CAD build for the part. Positions are in the model's coordinates, mm. Face numbers are marked on the shaded views. Round coordinates to 2 decimals unless told otherwise and drop trailing zeros. Loops run counter-clockwise (first coordinate to the right, second up) from the corner with the lowest first, then second, coordinate; pieces in that order, holes last. Notation, with made-up numbers: (-9, 41) -> (42, 41) arc R27 ccw to (42, 64) -> close; hole circle Ø9 at (-29, 35). An arc over 180 degrees is marked (long way). Answer as CSV lines item,"result".
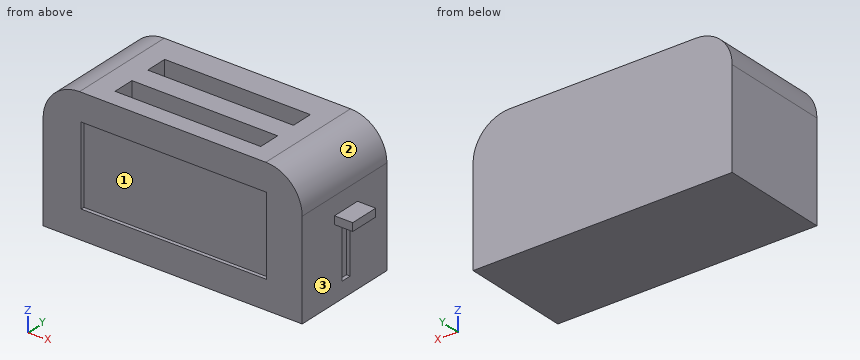
```python
from build123d import *

# Parameters (mm, degrees)
F0_W      = 180.69154
F0_H      = 93.475536
F1_DEPTH  = 76.2
F2_R      = 25.4
F3_W      = 101.6
F3_H      = 15.24
F4_DEPTH  = 76.2
F5_W      = 129.371017
F5_H      = 55.014919
F6_DEPTH  = 2.54
F7_W      = 20.702834
F7_H      = 5.605837
F8_DEPTH  = 12.7
F9_W      = 7.488246
F9_H      = 38.76276
F10_DEPTH = 2.54


with BuildPart() as f1:
    # F0 (on Front) → F1 (new body)
    with BuildSketch(Plane.XZ):
        with Locations((0, -8.763328)):
            Rectangle(F0_W, F0_H)
    extrude(amount=F1_DEPTH)

    # F2
    f2_edges = [f1.edges().sort_by_distance(p)[0] for p in [
        (90.34577, -38.1, 37.97444),
        (-90.34577, -38.1, 37.97444),
    ]]
    fillet(f2_edges, radius=F2_R)

    # F3 (on face) → F4 (cut)
    with BuildSketch(Plane.XY.offset(37.97444)):
        with Locations((1.085338, -56.274154)):
            Rectangle(F3_W, F3_H)
        with Locations((0.680554, -26.320373)):
            Rectangle(F3_W, F3_H)
    extrude(amount=-F4_DEPTH, mode=Mode.SUBTRACT)

    # F5 (on face) → F6 (cut)
    with BuildSketch(Plane.XZ.offset(76.2)):
        with Locations((0.859611, -8.333524)):
            Rectangle(F5_W, F5_H)
    extrude(amount=-F6_DEPTH, mode=Mode.SUBTRACT)

    # F7 (on face) → F8 (join)
    with BuildSketch(Plane.YZ.offset(90.34577)):
        with Locations((-36.778546, -2.802919)):
            Rectangle(F7_W, F7_H)
    extrude(amount=F8_DEPTH)

    # F9 (on face) → F10 (cut)
    with BuildSketch(Plane.YZ.offset(90.34577)):
        with Locations((-36.778546, -24.987215)):
            Rectangle(F9_W, F9_H)
    extrude(amount=-F10_DEPTH, mode=Mode.SUBTRACT)


solid = f1.part
```
Q1. Slice it at A-A, the plane z = 6. Give the cut face in (x, y), and give its area (3 significant figures).
Results:
outline,"(-90.35, -76.2) -> (-63.83, -76.2) -> (-63.83, -73.66) -> (65.55, -73.66) -> (65.55, -76.2) -> (90.35, -76.2) -> (90.35, 0) -> (-90.35, 0) -> close; hole (-50.12, -33.94) -> (51.48, -33.94) -> (51.48, -18.7) -> (-50.12, -18.7) -> close; hole (-49.71, -63.89) -> (51.89, -63.89) -> (51.89, -48.65) -> (-49.71, -48.65) -> close"
area,"10,300 mm2"
Q2. Slice it at B-B, the plane y = -56. Give the cut face in (x, z), and give its area (3 significant figures).
Results:
outline,"(-90.35, -55.5) -> (90.35, -55.5) -> (90.35, 12.57) arc R25.4 ccw to (64.95, 37.97) -> (51.89, 37.97) -> (51.89, -38.23) -> (-49.71, -38.23) -> (-49.71, 37.97) -> (-64.95, 37.97) arc R25.4 ccw to (-90.35, 12.57) -> close"
area,"8,870 mm2"
Q3. Slice it at C-C, the plane x = 17. Give the cut face in (y, z), and give its area (3 significant figures).
Results:
outline,"(-76.2, -55.5) -> (0, -55.5) -> (0, 37.97) -> (-18.7, 37.97) -> (-18.7, -38.23) -> (-33.94, -38.23) -> (-33.94, 37.97) -> (-48.65, 37.97) -> (-48.65, -38.23) -> (-63.89, -38.23) -> (-63.89, 37.97) -> (-76.2, 37.97) -> (-76.2, 19.17) -> (-73.66, 19.17) -> (-73.66, -35.84) -> (-76.2, -35.84) -> close"
area,"4,660 mm2"
Q4. Probe L1, parallel to Y at x = -10, z = 29; L2, parallel to Y at x = -32.5, z = 5; L3, parallel to X at y = -50, z = 4. List the from-to ranges inside material, lowest first. Write a range as [from, to].
Results:
L1,"[-76.2, -63.89], [-48.65, -33.94], [-18.7, 0]"
L2,"[-73.66, -63.89], [-48.65, -33.94], [-18.7, 0]"
L3,"[-90.35, -49.71], [51.89, 90.35]"
Q5. Drop flat-ended pins along their axis: pin 1 Ø7.5 at (y, z) = (-25.5, 15) entering from +X; pin 2 Ø1.7 at (x, z) = (98.5, -2) entering from +Y; pin 3 Ø10 at (x, y) = (96, -40.5) entering from +Z. Give the stop position or say it passes through.
Results:
pin 1,"x = 90.35"
pin 2,"y = -26.43"
pin 3,"z = 0"
Q6. Two-plate mould, pull along Z, no slides. Class the marked faces 1, 2 and 3: pulls with the +Z half, pulls with the -Z half, needs draft (parallel to the pull), parting line crosses it, or undercut.
Results:
face 1,"undercut"
face 2,"pulls with the +Z half"
face 3,"needs draft"
Q7. Slice it at D-D, the plane z = 28. Give the cut face in (x, y), and give its area (3 significant figures).
Results:
outline,"(-85.13, -76.2) -> (85.13, -76.2) -> (85.13, 0) -> (-85.13, 0) -> close; hole (-50.12, -33.94) -> (51.48, -33.94) -> (51.48, -18.7) -> (-50.12, -18.7) -> close; hole (-49.71, -63.89) -> (51.89, -63.89) -> (51.89, -48.65) -> (-49.71, -48.65) -> close"
area,"9,880 mm2"
